For this review, use the dimensioned drawing (mm, ordinates from the lowest corner) and the shaded views. A direction names the side the tool comes from. Coordinates: 2 decimals unless noted, no trailing zeros. Order: outer loops, then holes, each group sorted by start corner. A loop starts at its lowest first (then second) coordinate and runs counter-clockwise, first axis right, second up. Notation, with made-up numbers: M -35,79.5 L -19,79.5 A24 ccw -19,101.5 Z; hole C 60.5,-6 d8. An arc over 180 degrees is marked long. Answer as CSV lines item,"result". Start each with the question number.
Q1. Consider section B-B on z = 16.5. Write out the cut boundary in (x, y), and give its area (3 significant figures).
Q2. Consider section D-D on y = 36. Write out the cut boundary in (x, z).
Q3. For P1, Ø1.5, axis at x = 28, z = 8.5, coming from the +Y side; P2, Ø2, axis at y = 96.5, z = 29.5, coming from the +X side; P3, Ø10, axis at x = 31, y = 16.5, coming from the +Z side, all flat-tipped, find the tip position at first contact; note any pin that passes through.
Q4. Consider section C-C on x = 9. Write out the cut boundary in (y, z), and give its area (3 significant figures).
Q5. Consider section A-A on y = 14. Write out the cut boundary in (x, z).
Q6. Wall thickness on L1, parallel to X at y = 77, z = 23; L2, parallel to Y at x = 12.5, z = 18.5; L3, parallel to Z at x = 2.5, y = 62.5: over which ranges is each line inside the solid? List them lowest first. Write a range as [from, to].
Q7. Machinability: for the marked faces 1, 2 and 3, which of the approach directions +Z, -Z, +X, -X, +Y, -Y give a long, thin tool a straight path to every point of the face, cutting with its end or side? Answer none if there is none.
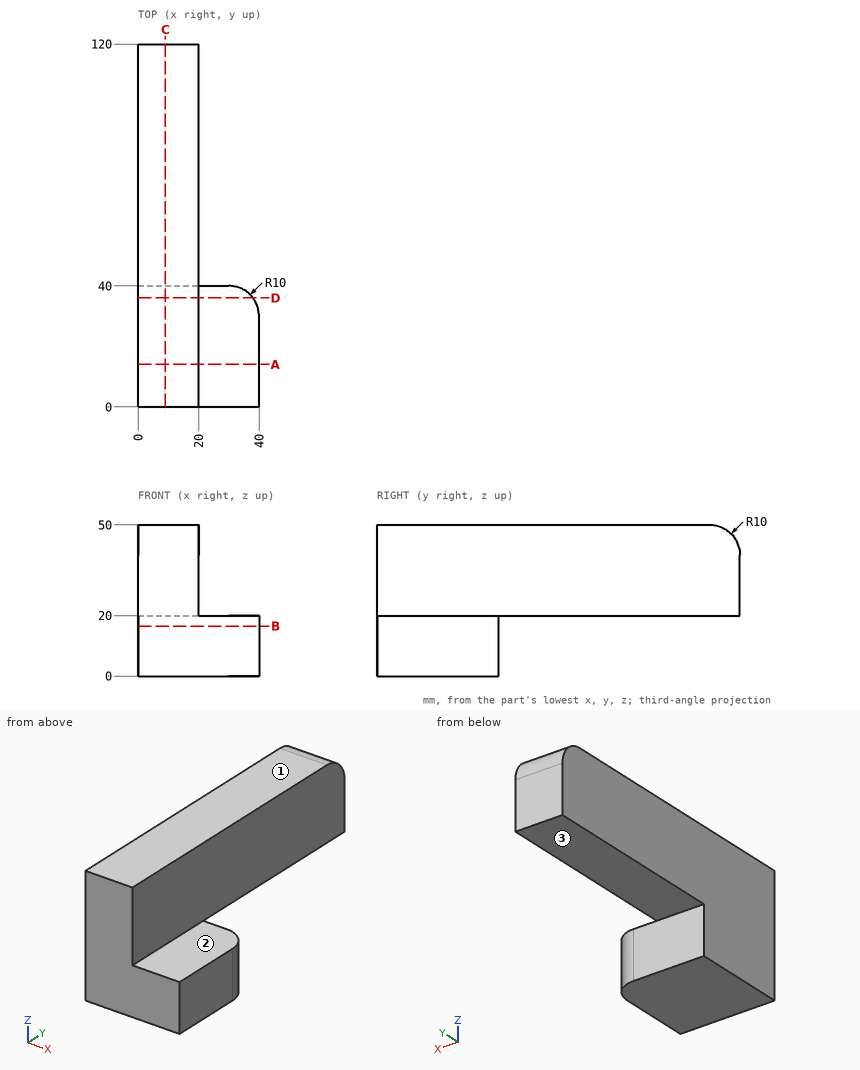
Evaluation:
1,outline,"M 0,0 L 40,0 L 40,30 A10 ccw 30,40 L 0,40 Z"
1,area,"1,580 mm²"
2,outline,"M 0,0 L 38,0 L 38,20 L 20,20 L 20,50 L 0,50 Z"
3,P1,"stops at y = 40"
3,P2,"stops at x = 20"
3,P3,"stops at z = 20"
4,outline,"M 0,0 L 40,0 L 40,20 L 120,20 L 120,40 A10 ccw 110,50 L 0,50 Z"
4,area,"4,380 mm²"
5,outline,"M 0,0 L 40,0 L 40,20 L 20,20 L 20,50 L 0,50 Z"
6,L1,"x = [0, 20]"
6,L2,"y = [0, 40]"
6,L3,"z = [20, 50]"
7,face 1,"+Z, +X, -X, +Y, -Y"
7,face 2,"+Z, +X, +Y, -Y"
7,face 3,"-Z, +X, -X, +Y"
